```python
from build123d import *

# Parameters (mm, degrees)
SKETCH1_R           = 50
BOSS_EXTRUDE1_DEPTH = 20
BOSS_EXTRUDE3_DEPTH = 30
BOSS_EXTRUDE7_DEPTH = 15
SKETCH5_R           = 2.5
CUT_EXTRUDE1_DEPTH  = 43
SKETCH8_R           = 7.5
CUT_EXTRUDE4_DEPTH  = 10
SKETCH9_R           = 2.5
CUT_EXTRUDE5_DEPTH  = 90
SKETCH10_R          = 12.5
CUT_EXTRUDE6_DEPTH  = 10
SKETCH11_R          = 15
BOSS_EXTRUDE8_DEPTH = 15
SKETCH12_R          = 10
CUT_EXTRUDE7_DEPTH  = 105


with BuildPart() as part:
    # Sketch1 → Boss-Extrude1 (new body)
    with BuildSketch(Plane.XY):
        Circle(SKETCH1_R)
    extrude(amount=BOSS_EXTRUDE1_DEPTH)

    # Sketch2 → Boss-Extrude3 (add)
    with BuildSketch(Plane.XY.offset(20)):
        with BuildLine():
            Line((-50, 0), (-45, 0))
            ThreePointArc((-45, 0), (0, -45), (45, 0))
            Line((45, 0), (50, 0))
            ThreePointArc((50, 0), (0, -50), (-50, 0))
        make_face()
    extrude(amount=BOSS_EXTRUDE3_DEPTH)

    # Sketch4 → Boss-Extrude7 (add)
    with BuildSketch(Plane.XY.offset(20)):
        with BuildLine():
            ThreePointArc((-48.989794856, 10), (-49.74680765, 5.0254481), (-50, 0))
            Line((-50, 0), (-45, 0))
            ThreePointArc((-45, 0), (0, -45), (45, 0))
            Line((45, 0), (50, 0))
            ThreePointArc((50, 0), (49.74680765, 5.0254481), (48.989794856, 10))
            ThreePointArc((48.989794856, 10), (21.419846516, 21.419846516), (10, 48.989794856))
            ThreePointArc((10, 48.989794856), (0, 50), (-10, 48.989794856))
            ThreePointArc((-10, 48.989794856), (-21.419846516, 21.419846516), (-48.989794856, 10))
        make_face()
    extrude(amount=BOSS_EXTRUDE7_DEPTH)

    # Sketch5 → Cut-Extrude1 (cut)
    with BuildSketch(Plane.XY.offset(20)):
        with Locations((-27.5, 27.5)):
            Circle(SKETCH5_R)
        with Locations((27.5, 27.5)):
            Circle(SKETCH5_R)
    extrude(amount=-CUT_EXTRUDE1_DEPTH, mode=Mode.SUBTRACT)

    # Sketch8 → Cut-Extrude4 (cut)
    with BuildSketch(Plane.XY.offset(35)):
        with Locations((0, -30)):
            Circle(SKETCH8_R)
    extrude(amount=-CUT_EXTRUDE4_DEPTH, mode=Mode.SUBTRACT)

    # Sketch9 → Cut-Extrude5 (cut)
    with BuildSketch(Plane.XY.offset(25)):
        with Locations((0, -30)):
            Circle(SKETCH9_R)
    extrude(amount=-CUT_EXTRUDE5_DEPTH, mode=Mode.SUBTRACT)

    # Sketch10 → Cut-Extrude6 (cut)
    with BuildSketch(Plane(origin=(0, 0, 0), x_dir=(-1, 0, 0), z_dir=(0, 0, -1))):
        with Locations((0, -30)):
            Circle(SKETCH10_R)
    extrude(amount=-CUT_EXTRUDE6_DEPTH, mode=Mode.SUBTRACT)

    # Sketch11 → Boss-Extrude8 (add)
    with BuildSketch(Plane.XY.offset(35)):
        Circle(SKETCH11_R)
    extrude(amount=BOSS_EXTRUDE8_DEPTH)

    # Sketch12 → Cut-Extrude7 (cut)
    with BuildSketch(Plane.XY.offset(50)):
        Circle(SKETCH12_R)
    extrude(amount=-CUT_EXTRUDE7_DEPTH, mode=Mode.SUBTRACT)


solid = part.part
```
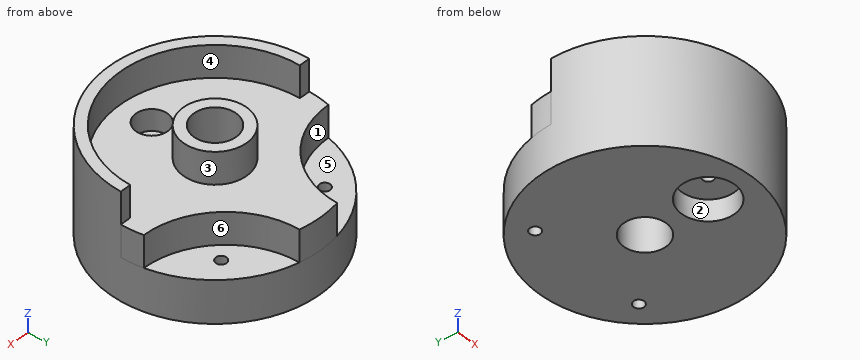
Geometry check sheet. Reference: the model listing, model coordinates, mm. Face numbers are marked on the shaded views. A direction names the side the tool comes from. Give positions to 0.01 mm unless a question says otherwise; leave off trailing zeros. Order: outer loops, then holes, each group sorted by start corner. A loop starts at its lowest first (then second) coordinate and runs counter-clockwise, first axis right, second up.
1. Release check for a two-part mould opening along Y. For the marked faces 4, 5 and 6 record: pulls with the +Y half, pulls with the -Y half, needs draft (parallel to the pull), parting line crosses it, or undercut.
2. Section check D-D, the plane z = 5.5. Enter the section's corners in (x, y), and give its area (3 significant figures).
3. Thickness scan on L1, parallel to Y at x = 0, z = 13; L2, parallel to Y at x = 0, z = 27.25; L3, parallel to Z at x = -13.5, y = -7.5. Record the ranges inside material, lowest first.
4. Section check B-B, the plane x = 0. Enter the section's corners in (y, z).
5. Gauge pin test, flat ends, axial feed: pin 1 Ø1 at (y, z) = (-14.5, 30) entering from +X; pin 2 Ø6.5 at (x, y) = (27.5, 27.5) entering from +Z; pin 3 Ø5 at (y, z) = (21, 25.5) entering from +X; pin 4 Ø12 at (x, y) = (0, 0) entering from -Z. Record the tip position at first contact, or that the pin passes through.
6. Section check C-C, the plane y = -30. Enter the section's corners in (x, z), and give its area (3 significant figures).
7. Access from +Z, -Z, +X, -X, +Y, -Y to the whole of each face (thin tool, end or side, straight path). Record for the marked faces 1, 2 and 3.
8. Section check A-A, the plane z = 44.5. Enter the section's corners in (x, y).
Values follow:
1. face 4: undercut
1. face 5: needs draft
1. face 6: pulls with the +Y half
2. outline: circle Ø100 at (0, 0); hole circle Ø5 at (-27.5, 27.5); hole circle Ø25 at (0, -30); hole circle Ø20 at (0, 0); hole circle Ø5 at (27.5, 27.5)
2. area: 7,010 mm2
3. L1: y = -50 to -32.5, -27.5 to -10, 10 to 50
3. L2: y = -50 to -37.5, -22.5 to -10, 10 to 50
3. L3: z = 0 to 35
4. outline: (-50, 0) - (-42.5, 0) - (-42.5, 10) - (-32.5, 10) - (-32.5, 25) - (-37.5, 25) - (-37.5, 35) - (-45, 35) - (-45, 50) - (-50, 50) - close; (-27.5, 10) - (-17.5, 10) - (-17.5, 0) - (-10, 0) - (-10, 50) - (-15, 50) - (-15, 35) - (-22.5, 35) - (-22.5, 25) - (-27.5, 25) - close; (10, 0) - (50, 0) - (50, 35) - (15, 35) - (15, 50) - (10, 50) - close
5. pin 1: stops at x = 48
5. pin 2: stops at z = 20
5. pin 3: stops at x = 24.69
5. pin 4: passes through
6. outline: (-40, 0) - (-12.5, 0) - (-12.5, 10) - (-2.5, 10) - (-2.5, 25) - (-7.5, 25) - (-7.5, 35) - (-33.54, 35) - (-33.54, 50) - (-40, 50) - close; (2.5, 10) - (12.5, 10) - (12.5, 0) - (40, 0) - (40, 50) - (33.54, 50) - (33.54, 35) - (7.5, 35) - (7.5, 25) - (2.5, 25) - close
6. area: 2,520 mm2
7. face 1: +Z, -X, +Y
7. face 2: -Z
7. face 3: +Z
8. outline: (-50, 0) arc R50 ccw to (50, 0) - (45, 0) arc R45 cw to (-45, 0) - close; circle Ø30 at (0, 0); hole circle Ø20 at (0, 0)
